Could you check a few things on this model? Use its own coordinates, in mm. A direction names the side the tool comes from. Give positions to 0.01 mm unless a question says otherwise; leave off trailing zeros. Order: outer loops, then holes, each group sorted by start corner. A loop starts at its lowest first (then second) coordinate and runs counter-clockwise, first axis right, second up. Notation, with made-up numbers: M -3.75,25 L 29.25,25 A12 ccw 29.25,38 Z; hole C 31,68 d9. An arc over 180 degrees is marked long. Use a Markdown table: item, result. Add a question column.
```python
from build123d import *

# Parameters (mm, degrees)
SKETCH1_W           = 23
SKETCH1_H           = 35
BOSS_EXTRUDE1_DEPTH = 0.78
SKETCH2_W           = 22
SKETCH2_H           = 17
BOSS_EXTRUDE2_DEPTH = 2.4
SKETCH3_W           = 3
SKETCH3_H           = 3
BOSS_EXTRUDE3_DEPTH = 1.75
SKETCH4_R           = 0.375
CUT_EXTRUDE1_DEPTH  = 1.78


with BuildPart() as part:
    # Sketch1 → Boss-Extrude1 (new body)
    with BuildSketch(Plane(origin=(0, 0, 0), x_dir=(1, 0, 0), z_dir=(0, 1, 0))):
        Rectangle(SKETCH1_W, SKETCH1_H)
    extrude(amount=BOSS_EXTRUDE1_DEPTH)

    # Sketch2 → Boss-Extrude2 (add)
    with BuildSketch(Plane(origin=(0, 0.78, 0), x_dir=(1, 0, 0), z_dir=(0, 1, 0))):
        with Locations((0, 3.5)):
            Rectangle(SKETCH2_W, SKETCH2_H)
    extrude(amount=BOSS_EXTRUDE2_DEPTH)

    # Sketch3 → Boss-Extrude3 (add)
    with BuildSketch(Plane(origin=(0, 0.78, 0), x_dir=(1, 0, 0), z_dir=(0, 1, 0))):
        with Locations((6.021341325, 14.744149298)):
            Rectangle(SKETCH3_W, SKETCH3_H)
    extrude(amount=BOSS_EXTRUDE3_DEPTH)

    # Sketch4 → Cut-Extrude1 (cut, through all)
    with BuildSketch(Plane(origin=(0, 0.78, 0), x_dir=(1, 0, 0), z_dir=(0, 1, 0))):
        with Locations((-9.736937967, -15.759105546)):
            Circle(SKETCH4_R)
        with Locations((-7.736937967, -15.759105546)):
            Circle(SKETCH4_R)
        with Locations((-5.736937967, -15.759105546)):
            Circle(SKETCH4_R)
        with Locations((-3.736937967, -15.759105546)):
            Circle(SKETCH4_R)
        with Locations((-1.736937967, -15.759105546)):
            Circle(SKETCH4_R)
        with Locations((0.263062033, -15.759105546)):
            Circle(SKETCH4_R)
        with Locations((2.263062033, -15.759105546)):
            Circle(SKETCH4_R)
        with Locations((-7.736937967, -13.759105546)):
            Circle(SKETCH4_R)
        with Locations((-5.736937967, -13.759105546)):
            Circle(SKETCH4_R)
        with Locations((-3.736937967, -13.759105546)):
            Circle(SKETCH4_R)
        with Locations((-1.736937967, -13.759105546)):
            Circle(SKETCH4_R)
        with Locations((0.263062033, -13.759105546)):
            Circle(SKETCH4_R)
        with Locations((2.263062033, -13.759105546)):
            Circle(SKETCH4_R)
        with Locations((-9.736937967, -13.759105546)):
            Circle(SKETCH4_R)
    extrude(amount=-CUT_EXTRUDE1_DEPTH, mode=Mode.SUBTRACT)


solid = part.part
```
1) Suppose I cut it at B-B on x = 5.5. Please give me the cut outline in (y, z).
2) Suppose I cut it at D-D on x = -1.75. Please give me the cut outline in (y, z).
3) Suppose I cut it at A-A on y = 1.5. Please give me the cut outline in (x, z).
4) For faces 4 (the face through (7.521, 2, -15)), 5 (the face through (6, 2, -16.244)), 6 (the face through (4.521, 2, -15)), 7 (the face through (-11, 2, -3)), which set-ups out of +Z, -Z, +X, -X, +Y, -Y let a thin tool reach every point of the face, with its end or its side?
5) Suppose I cut it at C-C on z = 4. Please give me the cut outline in (x, y).
6) We'd pull the mould along Z, two halves only. Please class faces 1 (the face through (6, 2, -13.244)), 2 (the face through (6, 2.53, -15)), 3 (the face through (0, 2, 5)): pulls with the +Z half, pulls with the -Z half, needs draft (parallel to the pull), parting line crosses it, or undercut.
7) For pin 1 (0.5 mm diameter, centred on y = 1.5, z = -14.5, fed in from -X); pin 2 (2.5 mm diameter, centred on x = 5.5, z = -14, fed in from +Y); pin 3 (0.7 mm diameter, centred on y = 1.5, z = -2.5, fed in from +X); pin 4 (1.9 mm diameter, centred on y = 1.5, z = -15.5, fed in from +X), each with a flat end and sliding along its axis, tell me the tip position at first contact or that it passes through.
8) Please list where these lines run through material, in increasing order: line 1 (Z direction, x = 5.5, y = 2.45); line 2 (Y direction, x = 9.75, z = 8.5); line 3 (X direction, y = 0.85, z = 0). Write a range as from..to.
Values found:
| question | item | result |
|---|---|---|
| 1 | outline | M 0,-17.5 L 0.78,-17.5 L 0.78,-16.24 L 2.53,-16.24 L 2.53,-13.24 L 0.78,-13.24 L 0.78,-12 L 3.18,-12 L 3.18,5 L 0.78,5 L 0.78,17.5 L 0,17.5 Z |
| 2 | outline | M 0,-17.5 L 0.78,-17.5 L 0.78,-12 L 3.18,-12 L 3.18,5 L 0.78,5 L 0.78,13.38 L 0,13.38 Z; M 0,14.13 L 0.78,14.13 L 0.78,15.38 L 0,15.38 Z; M 0,16.13 L 0.78,16.13 L 0.78,17.5 L 0,17.5 Z |
| 3 | outline | M -11,-12 L 11,-12 L 11,5 L -11,5 Z; M 4.52,-16.24 L 7.52,-16.24 L 7.52,-13.24 L 4.52,-13.24 Z |
| 4 | face 4 | -Z, +X, +Y |
| 4 | face 5 | -Z, +X, -X, +Y |
| 4 | face 6 | -Z, -X, +Y |
| 4 | face 7 | +Z, -Z, -X, +Y |
| 5 | outline | M -11.5,0 L 11.5,0 L 11.5,0.78 L 11,0.78 L 11,3.18 L -11,3.18 L -11,0.78 L -11.5,0.78 Z |
| 6 | face 1 | undercut |
| 6 | face 2 | needs draft |
| 6 | face 3 | pulls with the +Z half |
| 7 | pin 1 | stops at x = 4.52 |
| 7 | pin 2 | stops at y = 2.53 |
| 7 | pin 3 | stops at x = 11 |
| 7 | pin 4 | stops at x = 11.5 |
| 8 | line 1 | z = -16.24..-13.24, -12..5 |
| 8 | line 2 | y = 0..0.78 |
| 8 | line 3 | x = -11..11 |
